Study the drawing (mm; zero at the part's minimum x, y, z) and answer. Coordinates: 2 decimals unless noted, no trailing zeros. Loops run counter-clockwise (first coordinate to the right, second up) from the corner with the lowest first, then second, coordinate; pieces in that order, holes last. Notation, with made-up numbers: (30, 50.25) - (35, 50.25) arc R28 cw to (35, 75.25) - close; hole circle Ø3 at (-23, -25.75). An arc over 180 degrees is marked (long way). Use CSV: the item, a comma, the result in double quotes.
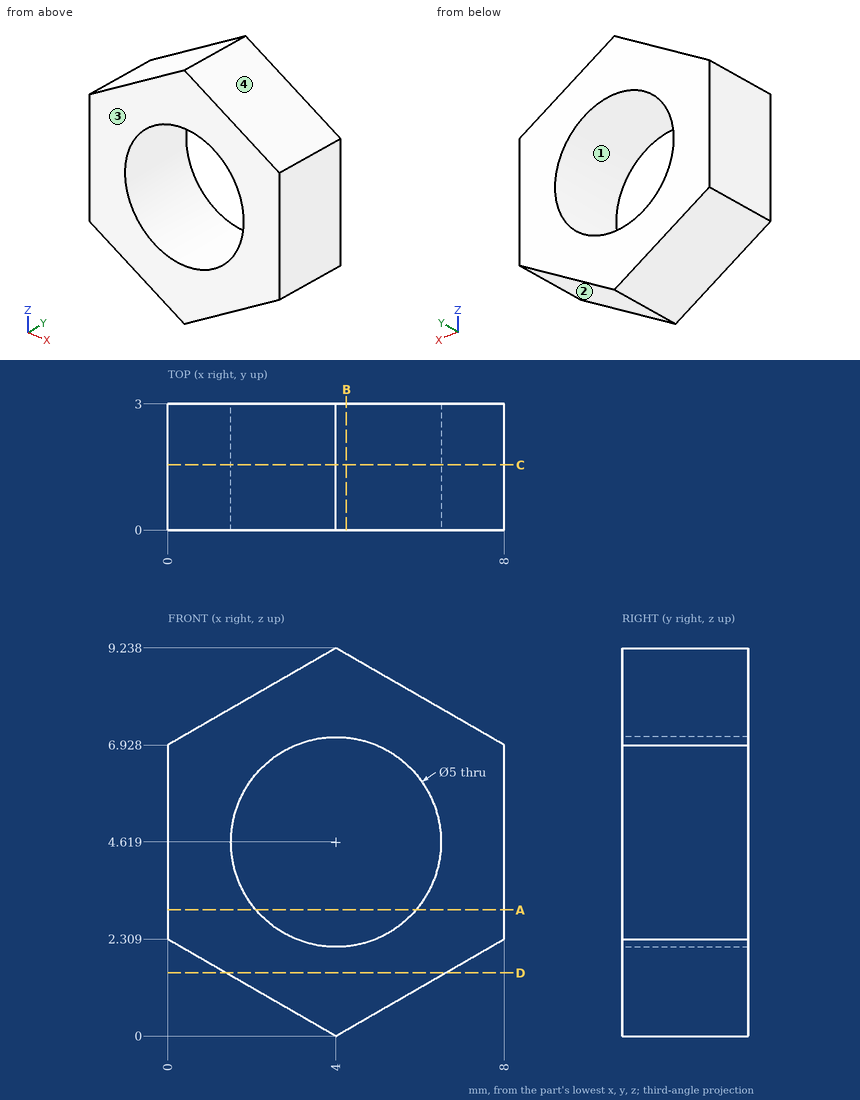
Q1. For a pull along Z with two mould halves and no side action, classify the marked faces 1, 2, 3 and 4 as +Z half, -Z half, draft (parallel to the pull), parting line (faces both ways), or undercut.
Reported:
face 1,"undercut"
face 2,"-Z half"
face 3,"draft"
face 4,"+Z half"
Q2. The part is cut by section A-A on z = 3. Determine the outline of the cut face in (x, y) (1 decimal), and give its area (3 significant figures).
Reported:
outline,"(0, 0) - (2.1, 0) - (2.1, 3) - (0, 3) - close; (5.9, 0) - (8, 0) - (8, 3) - (5.9, 3) - close"
area,"12.6 mm²"
Q3. The part is cut by section D-D on z = 1.5. Determine the outline of the cut face in (x, y).
Reported:
outline,"(1.4, 0) - (6.6, 0) - (6.6, 3) - (1.4, 3) - close"
Q4. Given P1, Ø1.5, axis at y = 1.5, z = 1.5, coming from the +X side (1 decimal); P2, Ø1.5, axis at x = 7, y = 2, coming from the -Z side, each flat-ended and moving along its own axis, determine where each tip first touches the part or whether it passes through.
Reported:
P1,"stops at x = 7.9"
P2,"stops at z = 1.3"
Q5. The part is cut by section C-C on y = 1.55. Determine the outline of the cut face in (x, z), and give its area (3 significant figures).
Reported:
outline,"(0, 2.31) - (4, 0) - (8, 2.31) - (8, 6.93) - (4, 9.24) - (0, 6.93) - close; hole circle Ø5 at (4, 4.62)"
area,"35.8 mm²"
Q6. Find the intervals of material crossed by probe 1 along X at (y, z) = (0.55, 4.5); probe 2 along Z at (x, y) = (5.5, 2.35) (1 decimal); probe 3 along X at (y, z) = (1.05, 5.5), in increasing order. Write a range as [from, to].
Reported:
probe 1,"x = [0, 1.5], [6.5, 8]"
probe 2,"z = [0.9, 2.6], [6.6, 8.4]"
probe 3,"x = [0, 1.66], [6.34, 8]"
Q7. The part is cut by section B-B on x = 4.25. Determine the outline of the cut face in (y, z) (1 decimal).
Reported:
outline,"(0, 0.1) - (3, 0.1) - (3, 2.1) - (0, 2.1) - close; (0, 7.1) - (3, 7.1) - (3, 9.1) - (0, 9.1) - close"
